from build123d import *

# Parameters (mm, degrees)
SKETCH_1_W                = 23.5
SKETCH_1_H                = 12
EXTRUDE_1_DEPTH           = 650.5
HOLE_WIZARD_M6_1_D        = 5
HOLE_WIZARD_M6_1_DEPTH    = 19
HOLE_WIZARD_M6_1_TIP      = 1.502151548
HOLE_WIZARD_M6_2_D        = 5
HOLE_WIZARD_M6_2_DEPTH    = 19
HOLE_WIZARD_M6_2_TIP      = 1.502151548
HOLE_WIZARD_9_0_9_1_D     = 9
HOLE_WIZARD_M6_3_D        = 5
HOLE_WIZARD_M6_3_DEPTH    = 15
HOLE_WIZARD_M6_3_TIP      = 1.502151548
HOLE_WIZARD_7_0_7_1_D     = 7
HOLE_WIZARD_7_0_7_1_DEPTH = 15
HOLE_WIZARD_7_0_7_1_TIP   = 2.103012167


with BuildPart() as part:
    # 草图1 → 凸台-拉伸1 (new, symmetric)
    with BuildSketch(Plane(origin=(0, 0, 0), x_dir=(0, 0, -1), z_dir=(1, 0, 0))):
        Polygon((-15, 15), (-11.5, 15), (-11.5, 13.5), (-11, 13.5), (-11, 12), (-9.5, 12), (-9.5, 15), (-8, 15), (-8, 12.5), (-5, 12.5), (-5, 15), (5, 15), (5, 12.5), (8, 12.5), (8, 15), (9.5, 15), (9.5, 12), (11, 12), (11, 13.5), (11.5, 13.5), (11.5, 15), (15, 15), (15, 8), (12.5, 8), (12.5, 5), (15, 5), (15, -5), (12.5, -5), (12.5, -8), (15, -8), (15, -15), (11.5, -15), (11.5, -13.5), (11, -13.5), (11, -12), (9.5, -12), (9.5, -15), (8, -15), (8, -12.5), (5, -12.5), (5, -15), (-5, -15), (-5, -12.5), (-8, -12.5), (-8, -15), (-9.5, -15), (-9.5, -12), (-11, -12), (-11, -13.5), (-11.5, -13.5), (-11.5, -15), (-15, -15), align=None)
        with BuildLine():
            Line((12, -10.5), (12, -8.5))
            ThreePointArc((12, -8.5), (11.853553391, -8.146446609), (11.5, -8))
            Line((11.5, -8), (-11.5, -8))
            ThreePointArc((-11.5, -8), (-11.853553391, -8.146446609), (-12, -8.5))
            Line((-12, -8.5), (-12, -10.5))
            ThreePointArc((-12, -10.5), (-11.853553391, -10.853553391), (-11.5, -11))
            Line((-11.5, -11), (11.5, -11))
            ThreePointArc((11.5, -11), (11.853553391, -10.853553391), (12, -10.5))
        make_face(mode=Mode.SUBTRACT)
        with BuildLine():
            Line((-11.5, 11), (11.5, 11))
            ThreePointArc((11.5, 11), (11.853553391, 10.853553391), (12, 10.5))
            Line((12, 10.5), (12, 8.5))
            ThreePointArc((12, 8.5), (11.853553391, 8.146446609), (11.5, 8))
            Line((11.5, 8), (-11.5, 8))
            ThreePointArc((-11.5, 8), (-11.853553391, 8.146446609), (-12, 8.5))
            Line((-12, 8.5), (-12, 10.5))
            ThreePointArc((-12, 10.5), (-11.853553391, 10.853553391), (-11.5, 11))
        make_face(mode=Mode.SUBTRACT)
        Rectangle(SKETCH_1_W, SKETCH_1_H, mode=Mode.SUBTRACT)
    extrude(amount=EXTRUDE_1_DEPTH, both=True)

    # M6 螺纹孔1
    with Locations(Plane(origin=(0, 15, 0), x_dir=(1, 0, 0), z_dir=(0, 1, 0))):
        with Locations((630.5, 0), (615.5, 0), (-630.5, 0), (-615.5, 0)):
            Hole(HOLE_WIZARD_M6_1_D / 2, depth=HOLE_WIZARD_M6_1_DEPTH)
            with Locations((0, 0, -(HOLE_WIZARD_M6_1_DEPTH + HOLE_WIZARD_M6_1_TIP / 2))):  # 118° drill point
                Cone(0, HOLE_WIZARD_M6_1_D / 2, HOLE_WIZARD_M6_1_TIP, mode=Mode.SUBTRACT)

    # M6 螺纹孔2
    with Locations(Plane(origin=(0, 0, -15), x_dir=(-1, 0, 0), z_dir=(0, 0, -1))):
        with Locations((-630.5, 0), (-615.5, 0), (615.5, 0), (630.5, 0)):
            Hole(HOLE_WIZARD_M6_2_D / 2, depth=HOLE_WIZARD_M6_2_DEPTH)
            with Locations((0, 0, -(HOLE_WIZARD_M6_2_DEPTH + HOLE_WIZARD_M6_2_TIP / 2))):  # 118° drill point
                Cone(0, HOLE_WIZARD_M6_2_D / 2, HOLE_WIZARD_M6_2_TIP, mode=Mode.SUBTRACT)

    # Ø9.0 (9) 直径孔1 (through all)
    with Locations(Plane.XY.offset(15)):
        with Locations((-525.5, 0), (-475.5, 0), (525.5, 0), (475.5, 0)):
            Hole(HOLE_WIZARD_9_0_9_1_D / 2)

    # M6 螺纹孔3
    with Locations(Plane(origin=(0, -15, 0), x_dir=(-1, 0, 0), z_dir=(0, -1, 0))):
        with Locations((425.5, 0), (0, 0), (-425.5, 0)):
            Hole(HOLE_WIZARD_M6_3_D / 2, depth=HOLE_WIZARD_M6_3_DEPTH)
            with Locations((0, 0, -(HOLE_WIZARD_M6_3_DEPTH + HOLE_WIZARD_M6_3_TIP / 2))):  # 118° drill point
                Cone(0, HOLE_WIZARD_M6_3_D / 2, HOLE_WIZARD_M6_3_TIP, mode=Mode.SUBTRACT)

    # Ø7.0 (7) 直径孔1
    with Locations(Plane(origin=(0, 15, 0), x_dir=(1, 0, 0), z_dir=(0, 1, 0))):
        with Locations((425.5, 0), (0, 0), (-425.5, 0)):
            Hole(HOLE_WIZARD_7_0_7_1_D / 2, depth=HOLE_WIZARD_7_0_7_1_DEPTH)
            with Locations((0, 0, -(HOLE_WIZARD_7_0_7_1_DEPTH + HOLE_WIZARD_7_0_7_1_TIP / 2))):  # 118° drill point
                Cone(0, HOLE_WIZARD_7_0_7_1_D / 2, HOLE_WIZARD_7_0_7_1_TIP, mode=Mode.SUBTRACT)


solid = part.part
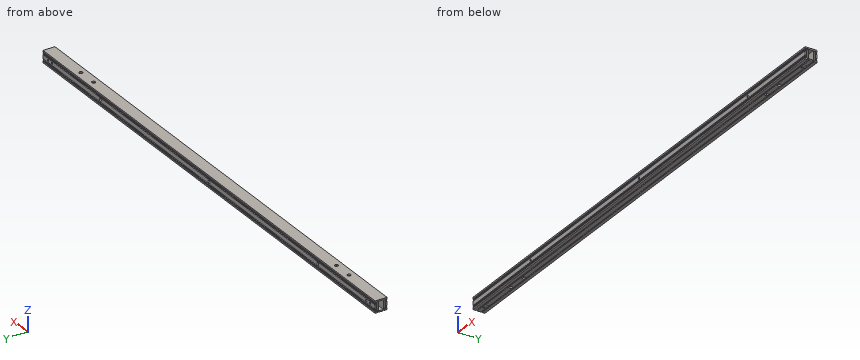
Could you check a few things on this model? Use its own coordinates, in mm. Give positions to 0.01 mm unless a question says otherwise; leave off trailing zeros. Answer as CSV lines item,"result". Start each with the question number.
(1) I'm going to push a flat-ended pin straight in: pin 1 Ø4.5 at (x, z) = (615.5, 0) entering from +Y. Where does the tip first touch, or does it pass through?
(2) If we section it at A-A, the plane x = 216.5: Give the number of separate pieces and of enclosed holes in the cut face, and give its area (3 significant figures).
(3) Please list where these lines run through material, in increasing order: line 1 (Y direction, x = -465.5, z = -10.75); line 2 (Y direction, x = -475.5, z = -13.8); line 3 (Z direction, x = -573, y = -13).
Answer list:
1,pin 1,"y = -6"
2,separate pieces,"1"
2,enclosed holes,"3"
2,area,"408 mm^2"
3,line 1,"-12 to -11, -8 to -6, 6 to 8, 11 to 12"
3,line 2,"-15 to -8, -5 to -4.5, 4.5 to 5, 8 to 15"
3,line 3,"-15 to -11, -9.5 to -8, -5 to 5, 8 to 9.5, 11 to 15"
